from build123d import *

# Parameters (mm, degrees)
SKETCH1_W           = 129
SKETCH1_H           = 209
BOSS_EXTRUDE1_DEPTH = 3.175
SKETCH2_R           = 1.25
SKETCH2_W           = 11
SKETCH2_H           = 25
CUT_EXTRUDE1_DEPTH  = 123.843724402
FILLET1_R           = 11
SKETCH3_R           = 1
CUT_EXTRUDE2_DEPTH  = 123.843724402
LPATTERN1_COUNT     = 2
LPATTERN1_PITCH     = 39
LPATTERN1_COL_COUNT = 2
LPATTERN1_COL_PITCH = 39
CUT_EXTRUDE3_DEPTH  = 123.843724402
SKETCH5_R           = 1.25
CUT_EXTRUDE4_DEPTH  = 123.843724402
SKETCH6_R           = 1.25
CUT_EXTRUDE5_DEPTH  = 123.843724402


with BuildPart() as part:
    # Sketch1 → Boss-Extrude1 (new body)
    with BuildSketch(Plane.XY):
        Rectangle(SKETCH1_W, SKETCH1_H)
    extrude(amount=BOSS_EXTRUDE1_DEPTH)

    # Sketch2 → Cut-Extrude1 (cut, through all)
    with BuildSketch(Plane.XY.offset(3.175)):
        with Locations((-59.5, 94.5)):
            Circle(SKETCH2_R)
        with Locations((-59.5, -74.5)):
            Circle(SKETCH2_R)
        with Locations(Location((59.5, -74.5, 0), (0, 0, 180))):
            Circle(SKETCH2_R)
        with Locations(Location((59.5, 94.5, 0), (0, 0, 180))):
            Circle(SKETCH2_R)
        with Locations((-59, -92)):
            Rectangle(SKETCH2_W, SKETCH2_H)
        with Locations((59, -92)):
            Rectangle(SKETCH2_W, SKETCH2_H)
    extrude(amount=-CUT_EXTRUDE1_DEPTH, mode=Mode.SUBTRACT)

    # Fillet1
    fillet1_edges = [part.edges().sort_by_distance(p)[0] for p in [
        (53.5, -79.5, 1.5875),
        (-53.5, -79.5, 1.5875),
    ]]
    fillet(fillet1_edges, radius=FILLET1_R - 0.0001)  # a hair under: the kernel refuses the full size

    # Sketch3 → Cut-Extrude2 (cut, through all)
    with BuildSketch(Plane.XY.offset(3.175)):
        with Locations((-10.25, 98.5)):
            Circle(SKETCH3_R)
        with Locations((10.25, 98.5)):
            Circle(SKETCH3_R)
        with Locations((-7.5, -43)):
            Circle(SKETCH3_R)
        with Locations((7.5, -43)):
            Circle(SKETCH3_R)
    cut_extrude2 = extrude(amount=-CUT_EXTRUDE2_DEPTH, mode=Mode.SUBTRACT)

    # LPattern1: Cut-Extrude2 ×2
    with Locations(*[(i * LPATTERN1_PITCH, 0, 0) for i in range(1, LPATTERN1_COUNT)]):
        add(cut_extrude2, mode=Mode.SUBTRACT)

    # LPattern1 col: Cut-Extrude2 ×2
    with Locations(*[(-i * LPATTERN1_COL_PITCH, 0, 0) for i in range(1, LPATTERN1_COL_COUNT)]):
        add(cut_extrude2, mode=Mode.SUBTRACT)

    # Sketch4 → Cut-Extrude3 (cut, through all)
    with BuildSketch(Plane.XY.offset(3.175)):
        with BuildLine():
            Line((-24.5, -104.5), (-24.5, -97))
            ThreePointArc((-24.5, -97), (-19.5, -92), (-14.5, -97))
            Line((-14.5, -97), (-14.5, -104.5))
            ThreePointArc((-14.5, -104.5), (-19.5, -109.5), (-24.5, -104.5))
        make_face()
        with BuildLine():
            Line((14.5, -104.5), (14.5, -97))
            ThreePointArc((14.5, -97), (19.5, -92), (24.5, -97))
            Line((24.5, -97), (24.5, -104.5))
            ThreePointArc((24.5, -104.5), (19.5, -109.5), (14.5, -104.5))
        make_face()
    extrude(amount=-CUT_EXTRUDE3_DEPTH, mode=Mode.SUBTRACT)

    # Sketch5 → Cut-Extrude4 (cut, through all)
    with BuildSketch(Plane.XY.offset(3.175)):
        with Locations((-10, 35.5)):
            Circle(SKETCH5_R)
        with Locations((-41.5, 35.5)):
            Circle(SKETCH5_R)
        with Locations((10, 35.5)):
            Circle(SKETCH5_R)
        with Locations((41.5, 35.5)):
            Circle(SKETCH5_R)
    extrude(amount=-CUT_EXTRUDE4_DEPTH, mode=Mode.SUBTRACT)

    # Sketch6 → Cut-Extrude5 (cut, through all)
    with BuildSketch(Plane(origin=(0, 0, 0), x_dir=(-1, 0, 0), z_dir=(0, 0, -1))):
        with Locations((-33.5, -22.5)):
            Circle(SKETCH6_R)
        with Locations((33.5, -22.5)):
            Circle(SKETCH6_R)
        with Locations((33.5, -64.5)):
            Circle(SKETCH6_R)
        with Locations((-33.5, -64.5)):
            Circle(SKETCH6_R)
    extrude(amount=-CUT_EXTRUDE5_DEPTH, mode=Mode.SUBTRACT)


solid = part.part
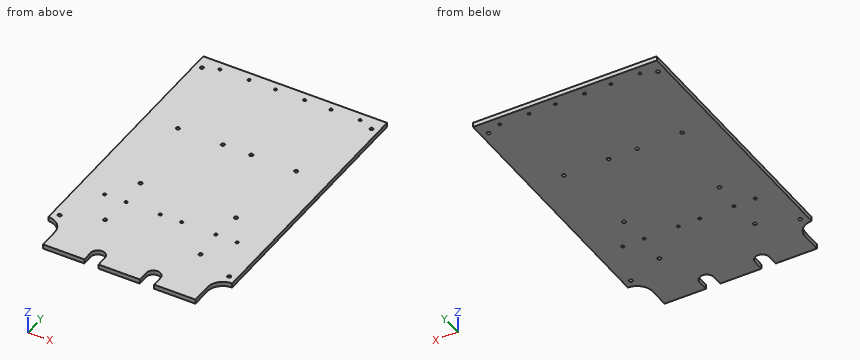
Can you work these out from the model? Positions are in its coordinate system, mm. Give positions to 0.01 mm unless a question says otherwise; leave off trailing zeros. Loops run counter-clockwise (first coordinate to the right, second up) from the corner with the lowest first, then second, coordinate; pieces in that order, holes last. Notation, with made-up numbers: (46, 84.5) -> (56, 84.5) arc R18 cw to (56, 108.5) -> close; hole circle Ø1 at (73.5, 64). An arc over 180 degrees is marked (long way). Return JSON: item names as keys, results as strings.
Q1. I want a section at A-A, the plane z = 2.35. Count the separate pieces of the cut face and the enclosed holes in it, then the cut area to 3 significant figures.
Checks:
{"separate pieces": "1", "enclosed holes": "24", "area": "26,100 mm2"}
Q2. I want a section at B-B, the plane x = 19.5. List the corners of the cut face in (y, z) for me (3 decimals).
Checks:
{"outline": "(-92, 0) -> (104.5, 0) -> (104.5, 3.175) -> (-92, 3.175) -> close"}
Q3. I want a section at C-C, the plane x = -55.5. List the corners of the cut face in (y, z) for me (3 decimals).
Checks:
{"outline": "(-84.175, 0) -> (104.5, 0) -> (104.5, 3.175) -> (-84.175, 3.175) -> close"}
Q4. I need wall thicknesses on probe 1 along Y at (x, z) = (-10, 0.2); probe 2 along Y at (x, z) = (-49.25, 2.05); probe 3 along Y at (x, z) = (9.5, 2.6). Which ranges of each line are inside material? Lowest first, please.
Checks:
{"probe 1": "y = -104.5 to 34.25, 36.75 to 97.53, 99.47 to 104.5", "probe 2": "y = -104.5 to 97.5, 99.5 to 104.5", "probe 3": "y = -104.5 to 34.35, 36.65 to 97.84, 99.16 to 104.5"}
Q5. For pin 1 Ø1 at (y, z) = (-100, 2) entering from +X; pin 2 Ø1.6 at (x, y) = (28.75, 98.5) entering from -Z, each with a flat end and sliding along its axis, tell me the tip position at first contact or that it passes through.
Checks:
{"pin 1": "stops at x = 53.5", "pin 2": "passes through"}
